Part model, mm, in its own coordinate system. A direction names the side the tool comes from. Round coordinates to 2 decimals unless told otherwise and drop trailing zeros. Loops run counter-clockwise (first coordinate to the right, second up) from the corner with the lowest first, then second, coordinate; pieces in that order, holes last. Notation, with made-up numbers: (-15, 49.5) -> (31, 49.5) arc R9 ccw to (31, 65.5) -> close; hole circle Ø9 at (30.5, -15). An arc over 180 degrees is marked (long way). Use a Markdown table: item, result. Add a question column.
Item 1: Which spindle directions (+Z, -Z, +X, -X, +Y, -Y) get a long thin tool onto all of the face, cutting with end or side? Do faces 4 (the face through (0, 53.672, 39)), 5 (the face through (6.35, 60, 35)), 6 (the face through (0, 60, 50.8)), 7 (the face through (-15, -54, 20.32)), 8 (the face through (-6.35, 60, 35)). Say none if no direction does.
Item 2: Probe line 1 (Z direction, x = 33.5, y = -36.5); line 2 (Z direction, x = -10, y = -57); line 3 (X direction, y = 57, z = 47). List the from-to ranges inside material, lowest first. Write a range as [from, to].
Item 3: Flat gauge pins, fed straight in: pin 1 (1 mm diameter, centred on x = -40, z = 14, fed in from -Y); pin 2 (8 mm diameter, centred on x = 6.5, y = 27, fed in from -Z); pin 3 (1 mm diameter, centred on x = -1.5, y = -31, fed in from +Z); pin 4 (6.5 mm diameter, centred on y = 61.5, z = 42.5, fed in from +X). Where does each tip first touch, or does it go through?
Item 4: Cut at D-D, the plane y = 37.5. List the corners of the cut face in (x, z).
Item 5: Cut at B-B, the plane y = 0. List the corners of the cut face in (x, z) (1 decimal), plus the area to 3 significant figures.
Item 6: Cut at C-C, the plane x = 18. List the corners of the cut face in (y, z), plus the area to 3 significant figures.
Item 7: Two-plate mould, pull along X, no slides. Class faces 1 (the face through (-41.42, 0.95, 39.19)), 2 (the face through (44, 0, 52.07)), 3 (the face through (-0.4, -41.3, 39.2)): pulls with the +X half, pulls with the -X half, needs draft (parallel to the pull), parting line crosses it, or undercut.
Item 8: Cut at A-A, the plane x = 0. List the corners of the cut face in (y, z) (1 decimal).
```python
from build123d import *

# Parameters (mm, degrees)
F1_DEPTH = 20.32
F3_DEPTH = 6.35
F5_DEPTH = 50.8
F6_R     = 3.175
F7_DEPTH = 25.4


with BuildPart() as f1:
    # F0 (on Top) → F1 (new body)
    with BuildSketch(Plane.XY):
        with BuildLine():
            Line((-6.35, 53.67193), (-6.35, 66.37193))
            ThreePointArc((-6.35, 66.37193), (0, -66.675), (6.35, 66.37193))
            Line((6.35, 66.37193), (6.35, 53.67193))
            Line((6.35, 53.67193), (-6.35, 53.67193))
        make_face()
    extrude(amount=F1_DEPTH)

    # F2 (on face) → F3 (join)
    with BuildSketch(Plane.XY.offset(20.32)):
        with BuildLine():
            Line((-6.35, 53.67193), (-6.35, 55.19845))
            ThreePointArc((-6.35, 55.19845), (0, -55.5625), (6.35, 55.19845))
            Line((6.35, 55.19845), (6.35, 53.67193))
            Line((6.35, 53.67193), (-6.35, 53.67193))
        make_face()
    extrude(amount=F3_DEPTH)

    # F4 (on Top) → F5 (join)
    with BuildSketch(Plane.XY):
        Polygon((-6.35, 55.19845), (-6.35, 53.67193), (6.35, 53.67193), (6.35, 66.37193), (-6.35, 66.37193), align=None)
    extrude(amount=F5_DEPTH)

    # F6 (on face) → F7 (join)
    with BuildSketch(Plane.XY.offset(26.67)):
        with Locations((44.45, 0)):
            Circle(F6_R)
        with Locations((0, -44.45)):
            Circle(F6_R)
        with Locations((-44.45, 0)):
            Circle(F6_R)
    extrude(amount=F7_DEPTH)


solid = f1.part
```
A:
| question | item | result |
|---|---|---|
| 1 | face 4 | +Z, +X, -X |
| 1 | face 5 | +Z, +X, +Y |
| 1 | face 6 | +Z, +X, -X, +Y |
| 1 | face 7 | +Z |
| 1 | face 8 | +Z, -X, +Y |
| 2 | line 1 | z = [0, 26.67] |
| 2 | line 2 | z = [0, 20.32] |
| 2 | line 3 | x = [-6.35, 6.35] |
| 3 | pin 1 | stops at y = -53.72 |
| 3 | pin 2 | stops at z = 0 |
| 3 | pin 3 | stops at z = 26.67 |
| 3 | pin 4 | stops at x = 6.35 |
| 4 | outline | (-55.13, 0) -> (55.13, 0) -> (55.13, 20.32) -> (41, 20.32) -> (41, 26.67) -> (-41, 26.67) -> (-41, 20.32) -> (-55.13, 20.32) -> close |
| 5 | outline | (-66.7, 0) -> (66.7, 0) -> (66.7, 20.3) -> (55.6, 20.3) -> (55.6, 26.7) -> (47.6, 26.7) -> (47.6, 52.1) -> (41.3, 52.1) -> (41.3, 26.7) -> (-41.3, 26.7) -> (-41.3, 52.1) -> (-47.6, 52.1) -> (-47.6, 26.7) -> (-55.6, 26.7) -> (-55.6, 20.3) -> (-66.7, 20.3) -> close |
| 5 | area | 3,740 mm^2 |
| 6 | outline | (-64.2, 0) -> (64.2, 0) -> (64.2, 20.32) -> (52.57, 20.32) -> (52.57, 26.67) -> (-52.57, 26.67) -> (-52.57, 20.32) -> (-64.2, 20.32) -> close |
| 6 | area | 3,280 mm^2 |
| 7 | face 1 | undercut |
| 7 | face 2 | needs draft |
| 7 | face 3 | parting line crosses it |
| 8 | outline | (-66.7, 0) -> (66.4, 0) -> (66.4, 50.8) -> (53.7, 50.8) -> (53.7, 26.7) -> (-41.3, 26.7) -> (-41.3, 52.1) -> (-47.6, 52.1) -> (-47.6, 26.7) -> (-55.6, 26.7) -> (-55.6, 20.3) -> (-66.7, 20.3) -> close |
